Work out the finished part from the listing and answer in its coordinate system (mm). Face numbers are marked on the shaded views. A direction names the side the tool comes from. Round coordinates to 2 decimals unless told otherwise and drop trailing zeros. Loops run counter-clockwise (first coordinate to the right, second up) from the corner with the lowest first, then second, coordinate; pieces in that order, holes last.
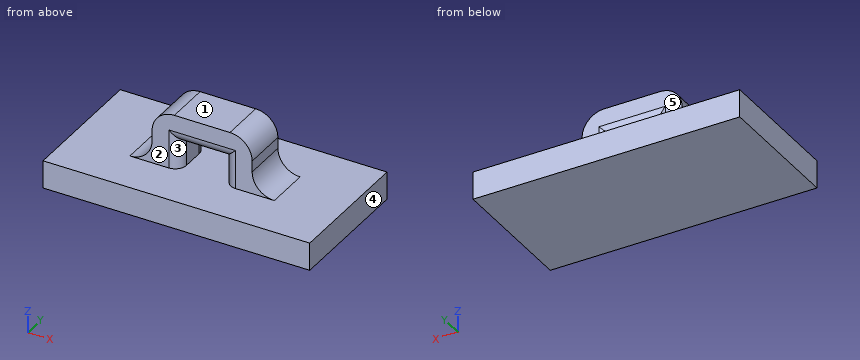
```python
from build123d import *

# Parameters (mm, degrees)
F0_W     = 24
F0_H     = 12
F1_DEPTH = 2.5
F3_DEPTH = 2
F4_R     = 2
F5_R     = 1


with BuildPart() as f1:
    # F0 (on Top) → F1 (new body)
    with BuildSketch(Plane.XY):
        Rectangle(F0_W, F0_H)
    extrude(amount=F1_DEPTH)

    # F2 (on Front) → F3 (join, symmetric)
    with BuildSketch(Plane.XZ):
        Polygon((4.5, 7.5), (-4.5, 7.5), (-4.5, 2.033843), (-2, 2.033843), (-2, 5), (2, 5), (2, 2.033843), (4.5, 2.033843), align=None)
    extrude(amount=F3_DEPTH, both=True)

    # F4
    f4_edges = [f1.edges().sort_by_distance(p)[0] for p in [
        (4.5, 0, 7.5),
        (-4.5, 0, 7.5),
        (4.5, 0, 2.5),
        (-4.5, 0, 2.5),
    ]]
    fillet(f4_edges, radius=F4_R)

    # F5
    f5_edges = [f1.edges().sort_by_distance(p)[0] for p in [
        (0, -2, 5),
        (0, 2, 5),
        (2, 2, 3.75),
        (-2, 2, 3.75),
        (2, -2, 3.75),
        (-2, -2, 3.75),
    ]]
    fillet(f5_edges, radius=F5_R)


solid = f1.part
```
1. Given pin 1 (1 mm diameter, centred on y = 0, z = 4.5, fed in from +X); pin 2 (2.5 mm diameter, centred on x = -2, z = 4, fed in from +Y); pin 3 (0.8 mm diameter, centred on y = 0, z = 5, fed in from -X), each flat-ended and moving along its own axis, determine where each tip first touches the part or whether it passes through.
Answer key:
pin 1: stops at x = 4.56
pin 2: stops at y = 2
pin 3: stops at x = -4.5
2. Which of the six approach directions +Z, -Z, +X, -X, +Y, -Y give full straight-line access (tool end or side, diameter ignored) to the marked faces 4 and 5?
Answer key:
face 4: +Z, -Z, +X, +Y, -Y
face 5: +Z, +X, -X, +Y
3. Find section C-C (z = 3). Write down the section's boundary in (x, y).
Answer key:
outline: (-5.18, -2) - (-3, -2) arc R1 ccw to (-2, -1) - (-2, 1) arc R1 ccw to (-3, 2) - (-5.18, 2) - close; (2, -1) arc R1 ccw to (3, -2) - (5.18, -2) - (5.18, 2) - (3, 2) arc R1 ccw to (2, 1) - close
4. Determine the mould class of the marked faces 1, 2 and 3 for opening direction Z: +Z half, -Z half, draft (parallel to the pull), parting line (faces both ways), or undercut.
Answer key:
face 1: +Z half
face 2: draft
face 3: undercut
5. Find section A-A (x = 0.5). Write down the section's boundary in (y, z).
Answer key:
outline: (-6, 0) - (6, 0) - (6, 2.5) - (-6, 2.5) - close; (-2, 6) arc R1 ccw to (-1, 5) - (1, 5) arc R1 ccw to (2, 6) - (2, 7.5) - (-2, 7.5) - close
6. Find section D-D (y = 2.5). Write down the section's boundary in (x, z).
Answer key:
outline: (-12, 0) - (12, 0) - (12, 2.5) - (-12, 2.5) - close
7. Find section B-B (y = -0.5). Write down the section's boundary in (x, z), then the cut area to 3 significant figures.
Answer key:
outline: (-12, 0) - (12, 0) - (12, 2.5) - (6.5, 2.5) arc R2 cw to (4.5, 4.5) - (4.5, 5.5) arc R2 ccw to (2.5, 7.5) - (-2.5, 7.5) arc R2 ccw to (-4.5, 5.5) - (-4.5, 4.5) arc R2 cw to (-6.5, 2.5) - (-12, 2.5) - close; hole (-2, 2.5) - (2, 2.5) - (2, 5) - (-2, 5) - close
area: 95.0 mm2
8. Consider probe 1 along Y at (x, z) = (-2, 6); probe 2 along Z at (x, y) = (10, 3); probe 3 along X at (y, z) = (0.25, 2.75). Determine where each line is inside the solid, lowest interval first.
Answer key:
probe 1: y = -2 to 2
probe 2: z = 0 to 2.5
probe 3: x = -5.53 to -2, 2 to 5.53
